The listing builds one solid part. Answer for the finished solid, in the listing's coordinates (mm). Face numbers are marked on the shaded views. A direction names the side the tool comes from. Give positions to 0.01 mm unless a question says otherwise; leave off trailing zeros. Write each loop counter-clockwise with the first axis right and the second up, starting at its lowest first coordinate (ties: lowest second). Pieces come first, ordered by that corner, then holes. Notation, with made-up numbers: M 17.25,55.25 L 59.25,55.25 A22 ccw 59.25,94.25 Z; hole C 8.5,-6 d9. An arc over 180 degrees is marked long. Return JSON: item names as keys, results as strings.
from build123d import *

# Parameters (mm, degrees)
SKETCH1_W           = 162.8
SKETCH1_H           = 122.8
SKETCH1_R           = 1.5
BOSS_EXTRUDE1_DEPTH = 6
FILLET1_R           = 6
SHELL5_T            = -3


with BuildPart() as part:
    # Sketch1 → Boss-Extrude1 (new body)
    with BuildSketch(Plane(origin=(0, 0, 0), x_dir=(1, 0, 0), z_dir=(0, 1, 0))):
        Rectangle(SKETCH1_W, SKETCH1_H)
        with Locations(Location((-74.100221616, 54.366983464, 0), (0, 0, 270))):
            Circle(SKETCH1_R, mode=Mode.SUBTRACT)
        with Locations(Location((74.107411227, 54.366983464, 0), (0, 0, 270))):
            Circle(SKETCH1_R, mode=Mode.SUBTRACT)
        with Locations(Location((74.107411227, -51.150377924, 0), (0, 0, 270))):
            Circle(SKETCH1_R, mode=Mode.SUBTRACT)
        with Locations(Location((-74.100221616, -51.150377924, 0), (0, 0, 270))):
            Circle(SKETCH1_R, mode=Mode.SUBTRACT)
    extrude(amount=BOSS_EXTRUDE1_DEPTH)

    # Fillet1
    fillet1_edges = [part.edges().sort_by_distance(p)[0] for p in [
        (81.4, 3, 61.4),
        (-81.4, 3, 61.4),
        (-81.4, 3, -61.4),
        (81.4, 3, -61.4),
    ]]
    fillet(fillet1_edges, radius=FILLET1_R)

    # Shell5
    shell5_openings = [part.faces().sort_by_distance(p)[0] for p in [
        (-5.099e-06, 6, 0.002281365),
    ]]
    offset(amount=SHELL5_T, openings=shell5_openings)


solid = part.part
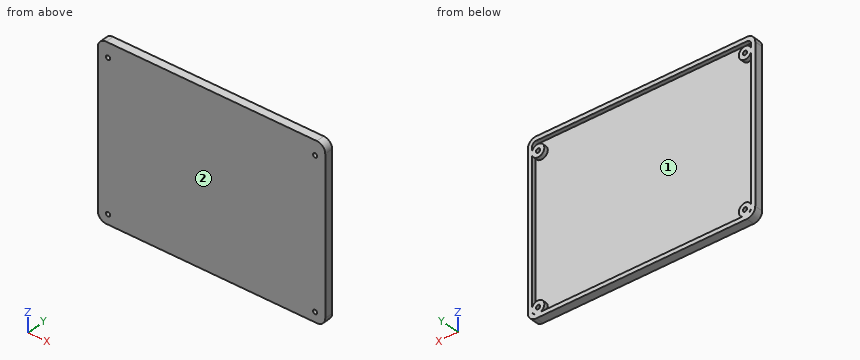
Item 1: A cutting plane is placed at A-A, the plane x = 22. Write down the section's boundary in (y, z).
Geometry results:
{"outline": "M 0,-61.4 L 6,-61.4 L 6,-58.4 L 3,-58.4 L 3,58.4 L 6,58.4 L 6,61.4 L 0,61.4 Z"}
Item 2: Which of the six approach directions +Z, -Z, +X, -X, +Y, -Y give full straight-line access (tool end or side, diameter ignored) to the marked faces 1 and 2?
Geometry results:
{"face 1": "+Y", "face 2": "+Z, -Z, +X, -X, -Y"}
Item 3: A cutting plane is placed at C-C, the plane y = 4.2. Write down the section's boundary in (x, z).
Geometry results:
{"outline": "M -81.4,-55.4 A6 ccw -75.4,-61.4 L 75.4,-61.4 A6 ccw 81.4,-55.4 L 81.4,55.4 A6 ccw 75.4,61.4 L -75.4,61.4 A6 ccw -81.4,55.4 Z; hole M -78.4,-53.04 A4.5 cw long -72.1,-58.4 L 72.11,-58.4 A4.5 cw long 78.4,-53.02 L 78.4,49.8 A4.5 cw long 78.4,52.5 L 78.4,55.4 A3 ccw 75.4,58.4 L -75.4,58.4 A3 ccw -78.4,55.4 L -78.4,52.48 A4.5 cw long -78.4,49.82 Z; hole M -78.38,-55.76 A3 ccw -76.43,-58.22 A4.5 cw Z; hole C -74.1,-54.37 d3; hole C -74.1,51.15 d3; hole C 74.11,-54.37 d3; hole C 74.11,51.15 d3; hole M 76.45,-58.21 A3 ccw 78.37,-55.8 A4.5 cw Z"}
Item 4: Given pin 1 Ø5 at (x, z) = (-16, -41) entering from +Y; pin 2 Ø2.5 at (x, z) = (-74.1, 51.15) entering from -Y, each flat-ended and moving along its own axis, determine where each tip first touches the part or whether it passes through.
Geometry results:
{"pin 1": "stops at y = 3", "pin 2": "passes through"}
Item 5: Find the intervals of material crossed by line 1 (X direction, y = 4.8, z = 18.5); line 2 (Z direction, x = 51, y = 3.45); line 3 (Y direction, x = 30.5, z = 46.5), in increasing order.
Geometry results:
{"line 1": "x = -81.4 to -78.4, 78.4 to 81.4", "line 2": "z = -61.4 to -58.4, 58.4 to 61.4", "line 3": "y = 0 to 3"}
Item 6: A cutting plane is placed at B-B, the plane z = 44. Write down the section's boundary in (x, y), plus the area to 3 significant figures.
Geometry results:
{"outline": "M -81.4,0 L 81.4,0 L 81.4,6 L 78.4,6 L 78.4,3 L -78.4,3 L -78.4,6 L -81.4,6 Z", "area": "506 mm2"}
